Here's the drawing with two shaded views (mm, measured from the low corner). I have some questions. Give positions to 0.01 mm unless a question says otherwise; leave off trailing zeros. Loops run counter-clockwise (first coordinate to the right, second up) from the corner with the lowest first, then second, coordinate; pieces in that order, holes last. Notation, with made-up numbers: (62, 40) -> (67, 40) arc R26 cw to (67, 66) -> close; hole circle Ø6 at (25.5, -29). An arc over 180 degrees is marked (long way). Answer in a Markdown table with one row per item. Add a question column.
Item 1: If we section it at B-B (x = 101.6): Write out the boundary of the cut face in (y, z).
Item 2: If we section it at A-A (y = 3.5): Write out the boundary of the cut face in (x, z), then the cut area to 3 significant figures.
Item 3: If we section it at C-C (z = 12.7): Write out the boundary of the cut face in (x, y).
Item 4: If I drill on line 1 (Z direction, x = 101.6, y = 4.5); line 2 (X direction, y = 2, z = 11.25); line 3 (X direction, y = 3, z = 9.5) (1 decimal), over which ranges is the centre line in solid material (lowest first)?
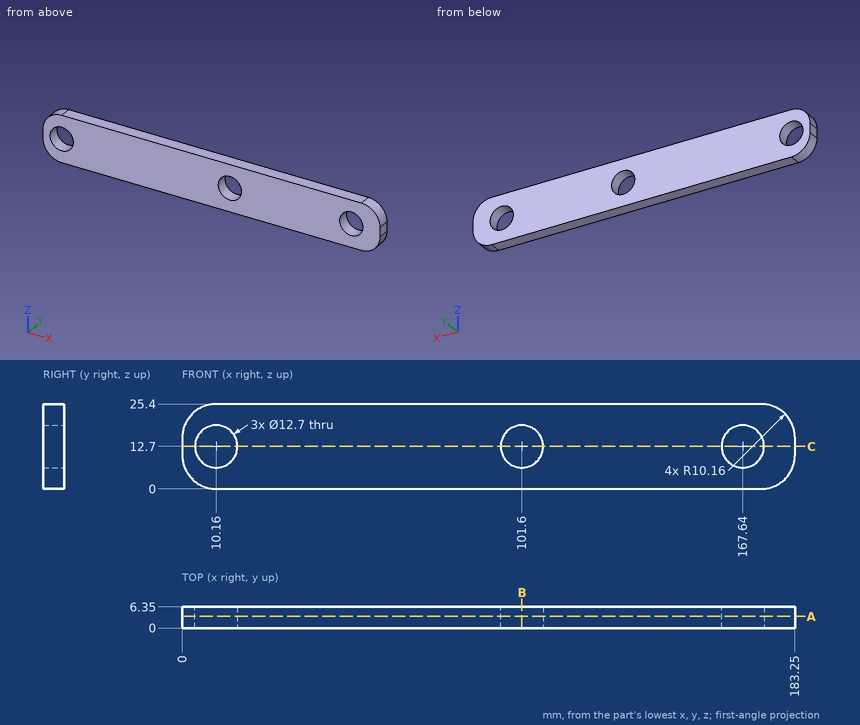
Recorded:
| question | item | result |
|---|---|---|
| 1 | outline | (0, 0) -> (6.35, 0) -> (6.35, 6.35) -> (0, 6.35) -> close; (0, 19.05) -> (6.35, 19.05) -> (6.35, 25.4) -> (0, 25.4) -> close |
| 2 | outline | (0, 10.16) arc R10.16 ccw to (10.16, 0) -> (173.09, 0) arc R10.16 ccw to (183.25, 10.16) -> (183.25, 15.24) arc R10.16 ccw to (173.09, 25.4) -> (10.16, 25.4) arc R10.16 ccw to (0, 15.24) -> close; hole circle Ø12.7 at (10.16, 12.7); hole circle Ø12.7 at (101.6, 12.7); hole circle Ø12.7 at (167.64, 12.7) |
| 2 | area | 4,190 mm^2 |
| 3 | outline | (0, 0) -> (3.81, 0) -> (3.81, 6.35) -> (0, 6.35) -> close; (16.51, 0) -> (95.25, 0) -> (95.25, 6.35) -> (16.51, 6.35) -> close; (107.95, 0) -> (161.29, 0) -> (161.29, 6.35) -> (107.95, 6.35) -> close; (173.99, 0) -> (183.25, 0) -> (183.25, 6.35) -> (173.99, 6.35) -> close |
| 4 | line 1 | z = 0 to 6.35, 19.05 to 25.4 |
| 4 | line 2 | x = 0 to 3.98, 16.34 to 95.42, 107.78 to 161.46, 173.82 to 183.25 |
| 4 | line 3 | x = 0 to 4.7, 15.6 to 96.1, 107.1 to 162.2, 173.1 to 183.2 |
